from build123d import *

# Parameters (mm, degrees)
F1_DEPTH = 381
F2_R     = 4.5
F3_DEPTH = 12.001
F4_R     = 2


with BuildPart() as f1:
    # F0 (on Right) → F1 (new body, symmetric)
    with BuildSketch(Plane.YZ):
        with BuildLine():
            Line((0, -11), (0, 0))
            Line((0, 0), (0, 11))
            ThreePointArc((0, 11), (-1.171573, 13.828427), (-4, 15))
            Line((-4, 15), (-8, 15))
            ThreePointArc((-8, 15), (-8.707107, 15.292893), (-9, 16))
            Line((-9, 16), (-9, 30))
            Line((-9, 30), (-12, 30))
            Line((-12, 30), (-12, 16))
            ThreePointArc((-12, 16), (-10.828427, 13.171573), (-8, 12))
            Line((-8, 12), (-4, 12))
            ThreePointArc((-4, 12), (-3.292893, 11.707107), (-3, 11))
            Line((-3, 11), (-3, 0))
            Line((-3, 0), (-3, -11))
            ThreePointArc((-3, -11), (-3.292893, -11.707107), (-4, -12))
            Line((-4, -12), (-8, -12))
            ThreePointArc((-8, -12), (-10.828427, -13.171573), (-12, -16))
            Line((-12, -16), (-12, -30))
            Line((-12, -30), (-9, -30))
            Line((-9, -30), (-9, -16))
            ThreePointArc((-9, -16), (-8.707107, -15.292893), (-8, -15))
            Line((-8, -15), (-4, -15))
            ThreePointArc((-4, -15), (-1.171573, -13.828427), (0, -11))
        make_face()
    extrude(amount=F1_DEPTH, both=True)

    # F2 (on face) → F3 (cut, through all)
    with BuildSketch(Plane(origin=(0, 0, 0), x_dir=(-1, 0, 0), z_dir=(0, 1, 0))):
        with Locations((-100, 0)):
            Circle(F2_R)
        with Locations((100, 0)):
            Circle(F2_R)
    extrude(amount=-F3_DEPTH, mode=Mode.SUBTRACT)

    # F4
    f4_edges = [f1.edges().sort_by_distance(p)[0] for p in [
        (-381, -10.5, 30),
        (-381, -10.5, -30),
        (381, -10.5, 30),
        (381, -10.5, -30),
    ]]
    fillet(f4_edges, radius=F4_R)


solid = f1.part
Can you work these out from the model? Positions are in its coordinate system, mm. A direction names the side the tool comes from. Coordinates: 2 decimals unless noted, no trailing zeros. Write each loop counter-clockwise with the first axis right and the second up, starting at its lowest first coordinate (ties: lowest second). Pieces come first, ordered by that corner, then holes. Notation, with made-up numbers: (29, 56.5) -> (74, 56.5) arc R16 ccw to (74, 63.5) -> close; hole circle Ø2 at (70, 86). An arc over 180 degrees is marked (long way). Write each question's results on one line, items separated by ' | '. Start each with the question number.
Q1. We'd pull the mould along Z, two halves only. Please class faces 3 (the face through (5, -3, 0)), 4 (the face through (5, -9, -23)): +Z half, -Z half, draft (parallel to the pull), parting line (faces both ways), or undercut.
Q2. Imagine slicing it at A-A (x = 11.5). Write out the boundary of the cut face in (y, z), then the cut area to 3 significant figures.
Q3. On a 3-axis mill with a long thin cutter (end or side, diameter ignored), from which of +Z, -Z, +X, -X, +Y, -Y can I reach the whole of each face in a straight line? I mean faces 1 (the face through (5, -9, 23)), 2 (the face through (5, 0, 0)). Say none if no direction works.
Q4. If I drill on probe 1 along Z at (x, y) = (261.5, -8.5); probe 2 along Y at (x, z) = (-205.5, -21); probe 3 along X at (y, z) = (-2.5, 2.5), over which ranges is the centre line in solid material (lowest first)?
Q5. I'm going to push flat-ended pins straight in: pin 1 (1 mm diameter, centred on x = -241.5, z = -15, fed in from -Y); pin 2 (5 mm diameter, centred on y = -10, z = 9, fed in from +X); pin 3 (4.5 mm diameter, centred on x = -110.5, y = -6, fed in from -Z); pin 4 (8 mm diameter, centred on x = 97, z = 20.5, fed in from +Y). Where does each tip first touch, or does it pass through?
Taken from the geometry:
1) face 3: undercut | face 4: draft
2) outline: (-12, -30) -> (-9, -30) -> (-9, -16) arc R1 cw to (-8, -15) -> (-4, -15) arc R4 ccw to (0, -11) -> (0, 11) arc R4 ccw to (-4, 15) -> (-8, 15) arc R1 cw to (-9, 16) -> (-9, 30) -> (-12, 30) -> (-12, 16) arc R4 ccw to (-8, 12) -> (-4, 12) arc R1 cw to (-3, 11) -> (-3, -11) arc R1 cw to (-4, -12) -> (-8, -12) arc R4 ccw to (-12, -16) -> close | area: 221 mm^2
3) face 1: +Z, +X, -X, +Y | face 2: +Z, -Z, +X, -X, +Y
4) probe 1: z = -15.13 to -12.03, 12.03 to 15.13 | probe 2: y = -12 to -9 | probe 3: x = -381 to -103.74, -96.26 to 96.26, 103.74 to 381
5) pin 1: stops at y = -11.97 | pin 2: passes through | pin 3: stops at z = -15.03 | pin 4: stops at y = -9
